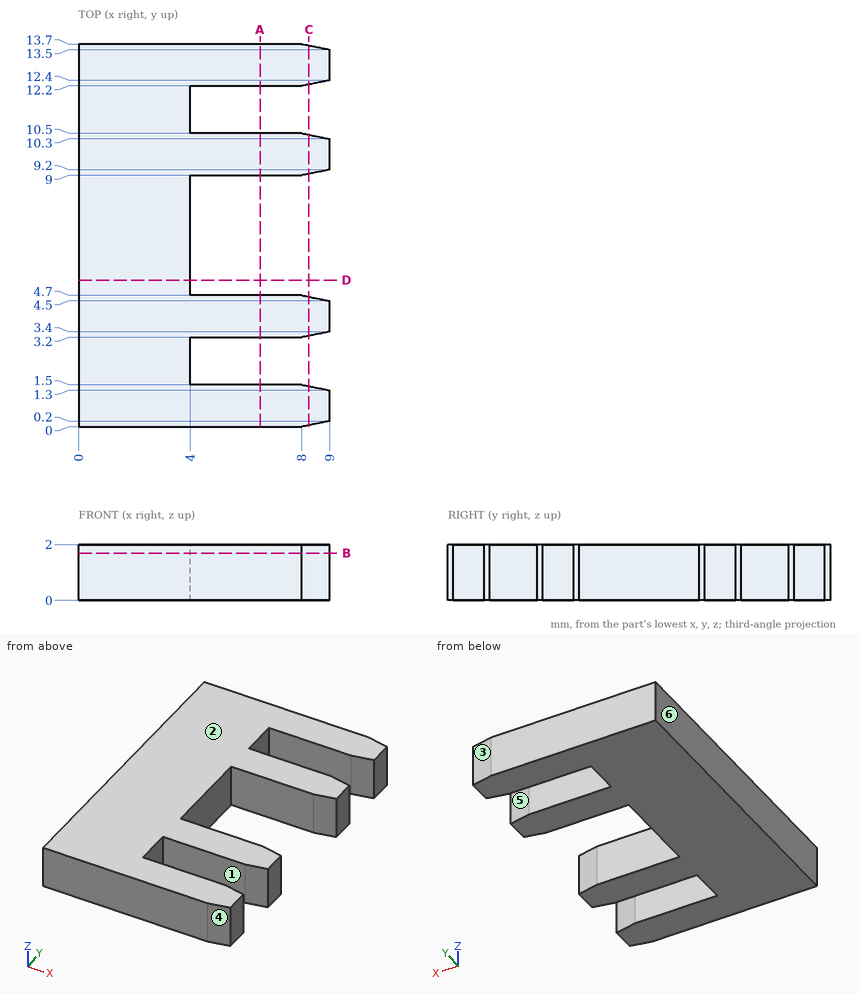
Geometry check sheet. Reference: drawing and pictorial views, mm from the part's lowest x, y, z. A direction names the side the tool comes from. Coordinates: 2 decimals unless noted, no trailing zeros. Order: outer loops, then holes, each group sorted by start corner. A loop starts at its lowest first (then second) coordinate and runs counter-clockwise, first axis right, second up. Notation, with made-up numbers: M 47,30.5 L 52,30.5 A22 ccw 52,45.5 Z; hole C 87.5,-30 d7. An arc over 180 degrees is marked long. Return JSON: item names as keys, results as strings.
1) Cross-section at B-B, the plane z = 1.7. Record the boundary of the cut face in (x, y), and give its area (3 significant figures).
Answer list:
{"outline": "M 0,0 L 8,0 L 9,0.2 L 9,1.3 L 8,1.5 L 4,1.5 L 4,3.2 L 8,3.2 L 9,3.4 L 9,4.5 L 8,4.7 L 4,4.7 L 4,9 L 8,9 L 9,9.2 L 9,10.3 L 8,10.5 L 4,10.5 L 4,12.2 L 8,12.2 L 9,12.4 L 9,13.5 L 8,13.7 L 0,13.7 Z", "area": "84.0 mm2"}
2) Cross-section at A-A, the plane x = 6.5. Record the boundary of the cut face in (y, z), and give its area (3 significant figures).
Answer list:
{"outline": "M 0,0 L 1.5,0 L 1.5,2 L 0,2 Z; M 3.2,0 L 4.7,0 L 4.7,2 L 3.2,2 Z; M 9,0 L 10.5,0 L 10.5,2 L 9,2 Z; M 12.2,0 L 13.7,0 L 13.7,2 L 12.2,2 Z", "area": "12.0 mm2"}
3) Thickness scan on L1, parallel to Y at x = 5.25, z = 0.6; L2, parallel to X at y = 6, z = 0.55. Record the ranges inside material, lowest first. Write a range as [from, to].
Answer list:
{"L1": "[0, 1.5], [3.2, 4.7], [9, 10.5], [12.2, 13.7]", "L2": "[0, 4]"}
4) Gauge pin test, flat end, axial feed: pin 1 (0.6 mm diameter, centred on y = 6, z = 0.5, fed in from +X). Record the tip position at first contact, or that the pin passes through.
Answer list:
{"pin 1": "x = 4"}
5) Cross-section at C-C, the plane x = 8.25. Record the boundary of the cut face in (y, z).
Answer list:
{"outline": "M 0.05,0 L 1.45,0 L 1.45,2 L 0.05,2 Z; M 3.25,0 L 4.65,0 L 4.65,2 L 3.25,2 Z; M 9.05,0 L 10.45,0 L 10.45,2 L 9.05,2 Z; M 12.25,0 L 13.65,0 L 13.65,2 L 12.25,2 Z"}
6) Release check for a two-part mould opening along Y. For the marked faces 3, 4, 5 and 6 record: +Y half, -Y half, draft (parallel to the pull), parting line (faces both ways), or undercut.
Answer list:
{"face 3": "+Y half", "face 4": "-Y half", "face 5": "undercut", "face 6": "draft"}
7) Cross-section at D-D, the plane y = 5.25. Record the boundary of the cut face in (x, z).
Answer list:
{"outline": "M 0,0 L 4,0 L 4,2 L 0,2 Z"}
8) Access from +Z, -Z, +X, -X, +Y, -Y to the whole of each face (thin tool, end or side, straight path). Record for the marked faces 1 and 2.
Answer list:
{"face 1": "+Z, -Z, +X", "face 2": "+Z, +X, -X, +Y, -Y"}
